Part model, mm, in its own coordinate system. Coordinates: 2 decimals unless noted, no trailing zeros. Loops run counter-clockwise (first coordinate to the right, second up) from the corner with the lowest first, then second, coordinate; pieces in that order, holes last. Notation, with made-up numbers: (33, -39) -> (57, -39) arc R26 cw to (57, -2) -> close; hole circle Ø10 at (4.25, -4.5). An arc over 180 degrees is marked (long way). Use one line per item in the form item = value. Start each with the question number.
(1) Band-saw the part on A-A on y = -13.5. Give the cut face in (x, z) (3 decimals), then the cut area to 3 significant figures.
(2) Mould opens along Y. For faces 1 (the flat face through (6, 0, 0)), 2 (the cylindrical face through (-24.78, -14.23, 4.7)), 3 (the cylindrical face through (22.9, 0.1, 4.7)) say: +Y half, -Y half, draft (parallel to the pull), parting line (faces both ways), or undercut.
(3) Pin check, flat tips, straight feed: P1, Ø3, axis at y = -18.5, z = 2.5, coming from the -X side; P2, Ø4, axis at x = 12.5, z = 6.5, coming from the -Y side; P3, Ø2, axis at x = -14.5, z = 2.5, coming from the -Y side. Stop position of each tip, or through.
(4) Band-saw the part on B-B on x = -13. Give the cut face in (y, z) (3 decimals).
(5) Band-saw the part on C-C on z = 8.75. Count the separate pieces of the cut face and the enclosed holes in it, then the cut area to 3 significant figures.
(6) Drill centre lines: L1, parallel to Y at x = 0, z = 4 (3 decimals); L2, parallel to X at y = 11.43, z = 5.75; L3, parallel to X at y = 22.86, z = 3.75. Where is each one in solid material? Low to high. Write a range as [from, to].
```python
from build123d import *

# Parameters (mm, degrees)
F0_R     = 28.575
F0_R_2   = 2.5
F1_DEPTH = 9.525
F3_DEPTH = 25.4
F4_R     = 0.5
F5_DEPTH = 25.4
F6_R     = 2


with BuildPart() as f1:
    # F0 (on Top) → F1 (new body)
    with BuildSketch(Plane.XY):
        Circle(F0_R)
        Circle(F0_R_2, mode=Mode.SUBTRACT)
    extrude(amount=F1_DEPTH)

    # F2 (on Top) → F3 (cut)
    with BuildSketch(Plane.XY):
        with BuildLine():
            ThreePointArc((6.6033751745, -33.3637991738), (17.0054966041, -29.4543841262), (25.592210064, -22.4005902387))
            ThreePointArc((25.592210064, -22.4005902387), (11.4492466041, -19.8306768266), (6.6033751745, -33.3637991738))
        make_face()
        with BuildLine():
            ThreePointArc((-25.592210064, -22.4005902387), (-17.0054966041, -29.4543841262), (-6.6033751745, -33.3637991738))
            ThreePointArc((-6.6033751745, -33.3637991738), (-6.0720335059, -31.4411002438), (-5.8929966041, -29.4543841262))
            ThreePointArc((-5.8929966041, -29.4543841262), (-13.259311683, -18.9923692731), (-25.592210064, -22.4005902387))
        make_face()
        with BuildLine():
            ThreePointArc((-22.8984932081, 0), (-25.5356944726, 7.187278177), (-32.1955852385, 10.9632089351))
            ThreePointArc((-32.1955852385, 10.9632089351), (-34.0109932081, 0), (-32.1955852385, -10.9632089351))
            ThreePointArc((-32.1955852385, -10.9632089351), (-25.5356944726, -7.187278177), (-22.8984932081, 0))
        make_face()
        with BuildLine():
            ThreePointArc((-5.8929966041, 29.4543841262), (-6.0720335059, 31.4411002438), (-6.6033751745, 33.3637991738))
            ThreePointArc((-6.6033751745, 33.3637991738), (-17.0054966041, 29.4543841262), (-25.592210064, 22.4005902387))
            ThreePointArc((-25.592210064, 22.4005902387), (-13.259311683, 18.9923692731), (-5.8929966041, 29.4543841262))
        make_face()
        with BuildLine():
            ThreePointArc((6.6033751745, 33.3637991738), (11.4492466041, 19.8306768266), (25.592210064, 22.4005902387))
            ThreePointArc((25.592210064, 22.4005902387), (17.0054966041, 29.4543841262), (6.6033751745, 33.3637991738))
        make_face()
        with BuildLine():
            ThreePointArc((32.1955852385, -10.9632089351), (33.5540719577, -5.55625), (34.0109932081, 0))
            ThreePointArc((34.0109932081, 0), (33.5540719577, 5.55625), (32.1955852385, 10.9632089351))
            ThreePointArc((32.1955852385, 10.9632089351), (22.8984932081, 0), (32.1955852385, -10.9632089351))
        make_face()
    extrude(amount=F3_DEPTH, mode=Mode.SUBTRACT)

    # F4 (on Top) → F5 (cut)
    with BuildSketch(Plane.XY):
        with Locations((0, 22.86)):
            Circle(F4_R)
        with Locations((-19.7973407305, 11.43)):
            Circle(F4_R)
        with Locations((-19.7973407305, -11.43)):
            Circle(F4_R)
        with Locations((0, -22.86)):
            Circle(F4_R)
        with Locations((19.7973407305, -11.43)):
            Circle(F4_R)
        with Locations((19.7973407305, 11.43)):
            Circle(F4_R)
    extrude(amount=F5_DEPTH, mode=Mode.SUBTRACT)

    # F6
    f6_edges = [f1.edges().sort_by_distance(p)[0] for p in [
        (-21.197157, 19.162755, 4.7625),
        (-5.996854, 27.938654, 4.7625),
        (21.197157, 19.162755, 4.7625),
        (5.996854, 27.938654, 4.7625),
        (-27.194011, -8.775899, 4.7625),
        (-27.194011, 8.775899, 4.7625),
        (-5.996854, -27.938654, 4.7625),
        (-21.197157, -19.162755, 4.7625),
        (21.197157, -19.162755, 4.7625),
        (5.996854, -27.938654, 4.7625),
        (27.194011, 8.775899, 4.7625),
        (27.194011, -8.775899, 4.7625),
    ]]
    fillet(f6_edges, radius=F6_R)


solid = f1.part
```
A:
q1.outline = (-25.185, 0) -> (25.185, 0) -> (25.185, 9.525) -> (-25.185, 9.525) -> close
q1.area = 480 mm²
q2.face_1 = draft
q2.face_2 = -Y half
q2.face_3 = undercut
q3.P1 = -22.97
q3.P2 = -20.45
q3.P3 = -18.91
q4.outline = (-19.089, 0) -> (19.089, 0) -> (19.089, 9.525) -> (-19.089, 9.525) -> close
q5.separate_pieces = 1
q5.enclosed_holes = 7
q5.area = 2,120 mm²
q6.L1 = [-28.575, -23.36], [-22.36, -2.5], [2.5, 22.36], [23.36, 28.575]
q6.L2 = [-26.19, -20.3], [-19.3, 19.3], [20.3, 26.19]
q6.L3 = [-8.06, -0.5], [0.5, 8.06]
